from build123d import *
from OCP.BRepFilletAPI import BRepFilletAPI_MakeFillet

# Parameters (mm, degrees)
SKETCH1_R                = 1.5
BOSS_EXTRUDE1_DEPTH      = 1.5
BOSS_EXTRUDE2_DEPTH      = 2
BOSS_EXTRUDE2_DEPTH_BACK = 1.5
SKETCH3_W                = 5
SKETCH3_H                = 0.7
SKETCH4_W                = 5
SKETCH4_H                = 1.5
BOSS_EXTRUDE3_DEPTH      = 0.15
FILLET2_R                = 0.85
SKETCH5_W                = 5
SKETCH5_H                = 1.2
BOSS_EXTRUDE4_DEPTH      = 2.5
BOSS_EXTRUDE4_2_DEPTH    = 2.5
SKETCH6_W                = 4
SKETCH6_H                = 5
BOSS_EXTRUDE5_DEPTH      = 2.35
FILLET3_R                = 1.5
CUT_EXTRUDE1_DEPTH       = 2.5
FILLET4_R1               = 3
FILLET4_R2               = 1
SKETCH8_W                = 5
SKETCH8_H                = 0.7
BOSS_EXTRUDE6_DEPTH      = 2
BOSS_EXTRUDE7_DEPTH      = 2


with BuildPart() as part:
    # Sketch1 → Boss-Extrude1 (new body)
    with BuildSketch(Plane(origin=(0, 0, 0), x_dir=(1, 0, 0), z_dir=(0, 1, 0))):
        with BuildLine():
            Line((0, 0), (60, 0))
            Line((60, 0), (60, 36))
            Line((60, 36), (60, 41))
            ThreePointArc((60, 41), (56, 45), (52, 41))
            Line((52, 41), (52, 36))
            Line((52, 36), (0, 36))
            Line((0, 36), (0, 0))
        make_face()
        with Locations(Location((56, 41, 0), (0, 0, 270))):
            Circle(SKETCH1_R, mode=Mode.SUBTRACT)
    extrude(amount=BOSS_EXTRUDE1_DEPTH)



with BuildPart() as body_2:
    # Sketch3 → Boss-Extrude2 (new, two sides: drawn at the far end of the back side and taken through both)
    with BuildSketch(Plane.XY.offset(-BOSS_EXTRUDE2_DEPTH_BACK)):
        with Locations((56, 2)):
            Rectangle(SKETCH3_W, SKETCH3_H)
    extrude(amount=BOSS_EXTRUDE2_DEPTH + BOSS_EXTRUDE2_DEPTH_BACK)


with BuildPart() as part_1:
    add(part.part)

    add(body_2.part)  # Boss-Extrude3 merges body 2
    # Sketch4 → Boss-Extrude3 (add)
    with BuildSketch(Plane.XZ.offset(-1.65)):
        with Locations((56, -0.75)):
            Rectangle(SKETCH4_W, SKETCH4_H)
    extrude(amount=BOSS_EXTRUDE3_DEPTH)

    # Fillet2
    fillet2_edges = [part_1.edges().sort_by_distance(p)[0] for p in [
        (56, 1.5, -1.5),
    ]]
    fillet(fillet2_edges, radius=FILLET2_R - 0.0001)  # a hair under: the kernel refuses the full size



with BuildPart() as body_2_2:
    # Sketch5 → Boss-Extrude4 (new body)
    with BuildSketch(Plane.ZY):
        with Locations((-10, 3.25)):
            Rectangle(SKETCH5_W, SKETCH5_H)
    extrude(amount=BOSS_EXTRUDE4_DEPTH)


with BuildPart() as body_3:
    # Sketch5 → Boss-Extrude4 2 (new body)
    with BuildSketch(Plane.ZY):
        with Locations((-26, 3.25)):
            Rectangle(SKETCH5_W, SKETCH5_H)
    extrude(amount=BOSS_EXTRUDE4_2_DEPTH)


with BuildPart() as part_2:
    add(part_1.part)

    add(body_2_2.part)  # Boss-Extrude5 merges body 2 2

    add(body_3.part)  # Boss-Extrude5 merges body 3
    # Sketch6 → Boss-Extrude5 (add)
    with BuildSketch(Plane(origin=(0, 1.5, 0), x_dir=(1, 0, 0), z_dir=(0, 1, 0))):
        with Locations((2, 26)):
            Rectangle(SKETCH6_W, SKETCH6_H)
        with Locations((2, 10)):
            Rectangle(SKETCH6_W, SKETCH6_H)
    extrude(amount=BOSS_EXTRUDE5_DEPTH)

    # Fillet3
    fillet3_edges = [part_2.edges().sort_by_distance(p)[0] for p in [
        (2, 1.5, -7.5),
    ]]
    fillet(fillet3_edges, radius=FILLET3_R)
    fillet3_2_edges = [part_2.edges().sort_by_distance(p)[0] for p in [
        (4, 1.5, -10),
    ]]
    fillet(fillet3_2_edges, radius=FILLET3_R)
    fillet3_3_edges = [part_2.edges().sort_by_distance(p)[0] for p in [
        (2, 1.5, -12.5),
    ]]
    fillet(fillet3_3_edges, radius=FILLET3_R)
    fillet3_4_edges = [part_2.edges().sort_by_distance(p)[0] for p in [
        (2, 1.5, -23.5),
    ]]
    fillet(fillet3_4_edges, radius=FILLET3_R)
    fillet3_5_edges = [part_2.edges().sort_by_distance(p)[0] for p in [
        (4, 1.5, -26),
    ]]
    fillet(fillet3_5_edges, radius=FILLET3_R - 0.0001)  # a hair under: the kernel refuses the full size
    fillet3_6_edges = [part_2.edges().sort_by_distance(p)[0] for p in [
        (2, 1.5, -28.5),
    ]]
    fillet(fillet3_6_edges, radius=FILLET3_R - 0.0001)  # a hair under: the kernel refuses the full size

    # Sketch7 → Cut-Extrude1 (cut)
    with BuildSketch(Plane(origin=(0, 1.5, 0), x_dir=(1, 0, 0), z_dir=(0, 1, 0))):
        Polygon((13.196152423, 29), (8, 32), (8, 26), align=None)
        Polygon((17, 26), (22.196152423, 29), (17, 32), align=None)
        Polygon((26, 26), (31.196152423, 29), (26, 32), align=None)
        Polygon((35, 26), (40.196152423, 29), (35, 32), align=None)
        Polygon((13.196152423, 18), (8, 21), (8, 15), align=None)
        Polygon((17, 15), (22.196152423, 18), (17, 21), align=None)
        Polygon((26, 15), (31.196152423, 18), (26, 21), align=None)
        Polygon((35, 15), (40.196152423, 18), (35, 21), align=None)
        Polygon((13.196152423, 7), (8, 10), (8, 4), align=None)
        Polygon((17, 4), (22.196152423, 7), (17, 10), align=None)
        Polygon((26, 4), (31.196152423, 7), (26, 10), align=None)
        Polygon((35, 4), (40.196152423, 7), (35, 10), align=None)
        Polygon((9.5, 23.5), (14.696152423, 26.5), (14.696152423, 20.5), align=None)
        Polygon((23.696152423, 20.5), (18.5, 23.5), (23.696152423, 26.5), align=None)
        Polygon((32.696152423, 20.5), (27.5, 23.5), (32.696152423, 26.5), align=None)
        Polygon((14.696152423, 9.5), (9.5, 12.5), (14.696152423, 15.5), align=None)
        Polygon((18.5, 12.5), (23.696152423, 15.5), (23.696152423, 9.5), align=None)
        Polygon((32.696152423, 9.5), (27.5, 12.5), (32.696152423, 15.5), align=None)
        Polygon((45, 26), (50.196152423, 29), (45, 32), align=None)
        Polygon((45, 15), (50.196152423, 18), (45, 21), align=None)
        Polygon((45, 4), (50.196152423, 7), (45, 10), align=None)
        Polygon((42.696152423, 20.5), (37.5, 23.5), (42.696152423, 26.5), align=None)
        Polygon((42.696152423, 9.5), (37.5, 12.5), (42.696152423, 15.5), align=None)
        Polygon((52.696152423, 20.5), (47.5, 23.5), (52.696152423, 26.5), align=None)
        Polygon((52.696152423, 9.5), (47.5, 12.5), (52.696152423, 15.5), align=None)
    extrude(amount=-CUT_EXTRUDE1_DEPTH, mode=Mode.SUBTRACT)

    # Fillet4: one fillet with a radius per group of edges: ONE call of the kernel's fillet builder (fillet() takes one radius for all edges)
    fillet4_edges_1 = [part_2.edges().sort_by_distance(p)[0] for p in [
        (0, 0.75, 0),
        (0, 0.75, -36),
    ]]
    fillet4_edges_2 = [part_2.edges().sort_by_distance(p)[0] for p in [
        (60, 0.75, 0),
    ]]
    fillet4 = BRepFilletAPI_MakeFillet(part_2.part.solid().wrapped)
    for e in fillet4_edges_1:
        fillet4.Add(FILLET4_R1, e.wrapped)
    for e in fillet4_edges_2:
        fillet4.Add(FILLET4_R2, e.wrapped)
    add(Compound.cast(fillet4.Shape()), mode=Mode.REPLACE)

    # Sketch8 → Boss-Extrude6 (add)
    with BuildSketch(Plane.XY.offset(2)):
        with Locations((56, 2)):
            Rectangle(SKETCH8_W, SKETCH8_H)
    extrude(amount=BOSS_EXTRUDE6_DEPTH)

    # Sketch9 → Boss-Extrude7 (add)
    with BuildSketch(Plane.ZY.offset(2.5)):
        with BuildLine():
            Line((-28.541404785, 2.65), (-23.458595215, 2.65))
            ThreePointArc((-23.458595215, 2.65), (-23.489612839, 2.823779714), (-23.5, 3))
            Line((-23.5, 3), (-23.5, 3.85))
            Line((-23.5, 3.85), (-28.5, 3.85))
            Line((-28.5, 3.85), (-28.5, 3))
            ThreePointArc((-28.5, 3), (-28.510387161, 2.823779714), (-28.541404785, 2.65))
        make_face()
        with BuildLine():
            Line((-12.541404785, 2.65), (-7.458595215, 2.65))
            ThreePointArc((-7.458595215, 2.65), (-7.489612839, 2.823779714), (-7.5, 3))
            Line((-7.5, 3), (-7.5, 3.85))
            Line((-7.5, 3.85), (-12.5, 3.85))
            Line((-12.5, 3.85), (-12.5, 3))
            ThreePointArc((-12.5, 3), (-12.510387161, 2.823779714), (-12.541404785, 2.65))
        make_face()
    extrude(amount=BOSS_EXTRUDE7_DEPTH)


solid = part_2.part
Input: part model. Units: mm. Frame: model coordinates. A direction names the side the tool comes from. Coordinates: 2 decimals unless noted, no trailing zeros. Loops run counter-clockwise (first coordinate to the right, second up) from the corner with the lowest first, then second, coordinate; pieces in that order, holes last.
(1) Pull-direction query (X, two-part tool) for faces 1 (the face through (0.86, 0.76, -35.1)), 2 (the face through (4.43, 1.95, -9.94)), 3 (the face through (28.6, 0.8, -27.5)); classes: released by +X, released by -X, zero draft, split by the parting line, or undercut.
(2) Section B-B on y = 0.65. Count the separate pieces of the cut face and the enclosed holes in it, then the cut area to 3 significant figures.
(3) Set-up query: faces 4 (the face through (37.6, 0.8, -16.5)), 5 (the face through (0, 3.85, -10)), 6 (the face through (-2, 2.65, -10)). Return all of +Z, -Z, +X, -X, +Y, -Y with unobstructed straight access to the full face (end or side cutting, diameter ignored); none if empty.
(4) Section C-C on z = 1. Return the cut outline in (x, y).
(5) Section D-D on z = -34. Return the cut outline in (x, y), then the cut area to 3 significant figures.
(6) Material intervals for probe 1 along X at (y, z) = (0.75, -41); probe 2 along X at (y, z) = (1.35, -20); probe 3 along Y at (x, z) = (53, -16), sorted ascending.
(7) First-contact query: pin 1 Ø1.2 at (y, z) = (1, -12.5) entering from -X; pin 2 Ø1.5 at (x, y) = (2, 1.5) entering from +Z; pin 3 Ø10 at (x, z) = (13, -4) entering from +Y. Flat tips, straight axial feed; report the tip coordinate or a pass-through.
Data:
1. face 1: released by -X
1. face 2: released by +X
1. face 3: undercut
2. separate pieces: 1
2. enclosed holes: 26
2. area: 1,820 mm2
3. face 4: +Y, -Y
3. face 5: +Z, -Z, +X, -X, +Y
3. face 6: +Z, -Z, -X, -Y
4. outline: (53.5, 1.65) - (58.5, 1.65) - (58.5, 2.35) - (53.5, 2.35) - close
5. outline: (0.17, 0) - (60, 0) - (60, 1.5) - (0.17, 1.5) - close
5. area: 89.7 mm2
6. probe 1: x = 52 to 54.5, 57.5 to 60
6. probe 2: x = 0 to 8, 9.73 to 17, 18.73 to 26, 27.73 to 35, 36.73 to 45, 46.73 to 60
6. probe 3: y = 0 to 1.5
7. pin 1: stops at x = 0
7. pin 2: stops at z = -0.01
7. pin 3: stops at y = 1.5
